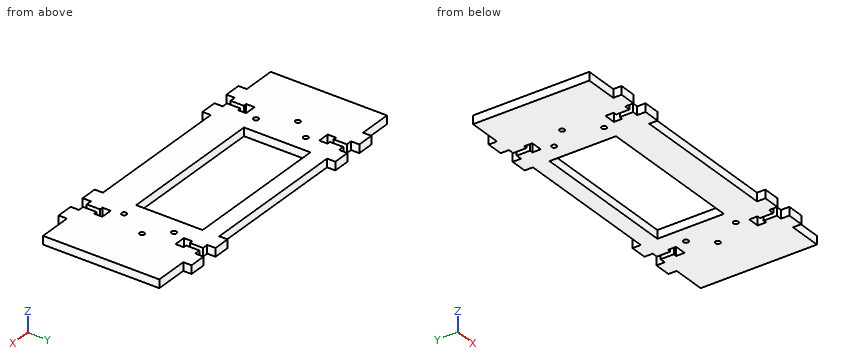
Autodesk Inventor part; units mm, degrees
ref_plane "YZ Plane" through (0, 0, 0) normal (1, 0, 0) x (0, 1, 0)
ref_plane "XZ Plane" through (0, 0, 0) normal (0, 1, 0) x (-1, 0, 0)
ref_plane "XY Plane" through (0, 0, 0) normal (0, 0, 1) x (1, 0, 0)
sketch "Sketch1" plane through (0, 0, 0) normal (0, 0, 1) x (1, 0, 0)
  line L0 (0, 0) -> (190, 0)
  line L1 (190, 0) -> (190, -70)
  line L2 (190, -70) -> (0, -70)
  line L3 (0, -70) -> (0, 0)
  line L4 (0, 0) -> (0, -40)
  line L5 (0, 0) -> (0, -10)
  line L6 (50, -10) -> (50, -50)
  line L7 (50, -50) -> (140, -50)
  line L8 (140, -50) -> (140, -10)
  line L9 (140, -10) -> (50, -10)
  circle A0 centre (40, -20) radius 1.5
  circle A1 centre (150, -20) radius 1.5
  circle A2 centre (150, -50) radius 1.5
  circle A3 centre (40, -50) radius 1.5
  line L10 (50, -10) -> (50, -12)
  line L11 (50, -12) -> (50, -32)
  line L12 (50, -32) -> (30, -32)
  line L13 (140, -32) -> (160, -32)
  circle A4 centre (30, -32) radius 1.5
  circle A5 centre (160, -32) radius 1.5
  dimension "d0" = 190
  dimension "d1" = 70
  dimension "d116" = 40
  dimension "d118" = 50
  dimension "d119" = 40
  dimension "d120" = 90
  dimension "d125" = 3
  dimension "d126" = 3
  dimension "d127" = 3
  dimension "d128" = 3
  dimension "d130" = 20
  dimension "d131" = 20
  dimension "d132" = 20
  dimension "d133" = 3
  dimension "d134" = 3
  dimension "d140" = 20
  dimension "d141" = 20
  dimension "d145" = 18
  dimension "d146" = 18
extrude "Extrusion3" add sketch "Sketch1" along normal blind 5 contours L0 L1 L2 L3 | L9 L8 L7 L6 | A5 | A4 | A0 | A1 | A2 | A3
sketch "Sketch3" plane through (0, 0, 0) normal (0, 0, -1) x (-1, 0, 0)
  line L0 (0, 0) -> (-35, 0)
  line L1 (-35, 0) -> (-35, -13)
  line L2 (-35, -13) -> (-31.5, -13)
  line L3 (-35, -13) -> (-38.5, -13)
  line L4 (-38.5, -13) -> (-38.5, -8)
  line L5 (-38.5, -8) -> (-36.5, -8)
  line L6 (-36.5, -8) -> (-36.5, 0)
  line L7 (-31.5, -13) -> (-31.5, -8)
  line L8 (-31.5, -8) -> (-33.5, -8)
  line L9 (-33.5, -8) -> (-33.5, 0)
  line L10 (-35, 0) -> (-75, 0) construction
  line L11 (-75, 0) -> (-75, -13)
  line L12 (-75, -13) -> (-71.5, -13)
  line L13 (-75, -13) -> (-78.5, -13)
  line L14 (-78.5, -13) -> (-78.5, -8)
  line L15 (-78.5, -8) -> (-76.5, -8)
  line L16 (-71.5, -13) -> (-71.5, -8)
  line L17 (-71.5, -8) -> (-73.5, -8)
  line L18 (-73.5, -8) -> (-73.5, 0)
  line L19 (-76.5, -8) -> (-76.5, 0)
  line L20 (0, 0) -> (-190, 0)
  line L21 (-75, 0) -> (-115, 0)
  line L22 (-115, 0) -> (-115, -13)
  line L23 (-115, -13) -> (-111.5, -13)
  line L24 (-111.5, -13) -> (-111.5, -8)
  line L25 (-111.5, -8) -> (-113.5, -8)
  line L26 (-113.5, -8) -> (-113.5, 0)
  line L27 (-115, -13) -> (-118.5, -13)
  line L28 (-118.5, -13) -> (-118.5, -8)
  line L29 (-118.5, -8) -> (-116.5, -8)
  line L30 (-116.5, -8) -> (-116.5, 0)
  line L31 (-115, 0) -> (-155, 0)
  line L32 (-155, 0) -> (-155, -13)
  line L33 (-155, -13) -> (-151.5, -13)
  line L34 (-151.5, -13) -> (-151.5, -8)
  line L35 (-151.5, -8) -> (-153.5, -8)
  line L36 (-153.5, -8) -> (-153.5, 0)
  line L37 (-155, -13) -> (-158.5, -13)
  line L38 (-158.5, -13) -> (-158.5, -8)
  line L39 (-158.5, -8) -> (-156.5, -8)
  line L40 (-156.5, -8) -> (-156.5, 0)
  line L41 (-76.5, 0) -> (-73.5, 0)
  line L42 (-33.5, -8) -> (-31.5, -8)
  line L43 (-36.5, 0) -> (-33.5, 0)
  line L44 (-155, 0) -> (-155, -70)
  line L45 (-115, 0) -> (-115, -70)
  line L46 (-75, 0) -> (-75, -70)
  line L47 (-35, 0) -> (-35, -70)
  line L48 (-155, -70) -> (-153.5, -70)
  line L49 (-153.5, -70) -> (-153.5, -62)
  line L50 (-153.5, -62) -> (-151.5, -62)
  line L51 (-151.5, -62) -> (-151.5, -57)
  line L52 (-151.5, -57) -> (-155, -57)
  line L53 (-155, -70) -> (-156.5, -70)
  line L54 (-156.5, -70) -> (-156.5, -62)
  line L55 (-156.5, -62) -> (-158.5, -62)
  line L56 (-158.5, -62) -> (-158.5, -57)
  line L57 (-158.5, -57) -> (-155, -57)
  line L58 (-115, -70) -> (-113.5, -70)
  line L59 (-113.5, -70) -> (-113.5, -62)
  line L60 (-113.5, -62) -> (-111.5, -62)
  line L61 (-111.5, -62) -> (-111.5, -57)
  line L62 (-111.5, -57) -> (-115, -57)
  line L63 (-115, -70) -> (-116.5, -70)
  line L64 (-116.5, -70) -> (-116.5, -62)
  line L65 (-116.5, -62) -> (-118.5, -62)
  line L66 (-118.5, -62) -> (-118.5, -57)
  line L67 (-118.5, -57) -> (-115, -57)
  line L68 (-75, -70) -> (-73.5, -70)
  line L69 (-73.5, -70) -> (-73.5, -62)
  line L70 (-73.5, -62) -> (-71.5, -62)
  line L71 (-71.5, -62) -> (-71.5, -57)
  line L72 (-71.5, -57) -> (-75, -57)
  line L73 (-75, -70) -> (-76.5, -70)
  line L74 (-76.5, -70) -> (-76.5, -62)
  line L75 (-76.5, -62) -> (-78.5, -62)
  line L76 (-78.5, -62) -> (-78.5, -57)
  line L77 (-78.5, -57) -> (-75, -57)
  line L78 (-35, -70) -> (-33.5, -70)
  line L79 (-33.5, -70) -> (-33.5, -62)
  line L80 (-33.5, -62) -> (-31.5, -62)
  line L81 (-31.5, -62) -> (-31.5, -57)
  line L82 (-31.5, -57) -> (-38.5, -57)
  line L83 (-38.5, -57) -> (-38.5, -62)
  line L84 (-38.5, -62) -> (-36.5, -62)
  line L85 (-36.5, -62) -> (-36.5, -70)
  line L86 (-36.5, -70) -> (-35, -70)
  dimension "d14" = 35
  dimension "d15" = 13
  dimension "d16" = 3.5
  dimension "d17" = 3.5
  dimension "d18" = 5
  dimension "d19" = 2
  dimension "d20" = 2
  dimension "d21" = 40
  dimension "d22" = 13
  dimension "d23" = 3.5
  dimension "d24" = 3.5
  dimension "d25" = 5
  dimension "d26" = 2
  dimension "d27" = 2
  dimension "d28" = 40
  dimension "d29" = 8
  dimension "d30" = 13
  dimension "d31" = 40
  dimension "d32" = 13
  dimension "d33" = 3.5
  dimension "d34" = 5
  dimension "d35" = 2
  dimension "d36" = 3.5
  dimension "d37" = 5
  dimension "d38" = 2
  dimension "d39" = 40
  dimension "d40" = 13
  dimension "d41" = 3.5
  dimension "d42" = 5
  dimension "d43" = 2
  dimension "d44" = 3.5
  dimension "d45" = 5
  dimension "d46" = 2
  dimension "d63" = 8
  dimension "d66" = 1.5
  dimension "d67" = 5
  dimension "d68" = 1.5
  dimension "d69" = 2
  dimension "d70" = 5
  dimension "d71" = 1.5
  dimension "d72" = 2
  dimension "d73" = 8
  dimension "d74" = 2
  dimension "d75" = 1.5
extrude "Extrusion4" cut sketch "Sketch3" against normal blind 5 contours L32 L37 L38 L39 L40 L20
extrude "Extrusion5" cut sketch "Sketch3" against normal blind 5 contours L36 L35 L34 L33 L32 L20
extrude "Extrusion9" cut sketch "Sketch3" against normal blind 5 contours L9 L8 L7 L2 L1 L0
extrude "Extrusion10" cut sketch "Sketch3" against normal blind 5 contours L1 L3 L4 L5 L6 L20
extrude "Extrusion11" cut sketch "Sketch3" against normal blind 5 contours L44 L53 L54 L55 L56 L57
extrude "Extrusion12" cut sketch "Sketch3" against normal blind 5 contours L52 L51 L50 L49 L48 L44
extrude "Extrusion17" cut sketch "Sketch3" against normal blind 5 contours L82 L81 L80 L79 L78 L47 | L47 L86 L85 L84 L83 L82
sketch "Sketch4" plane through (153.5, -70, 0) normal (0, -1, 0) x (1, 0, 0)
  line L0 (-153.5, 0) -> (-133.5, 0)
  line L1 (-133.5, 0) -> (-133.5, 5)
  line L2 (-133.5, 5) -> (-123.5, 5)
  line L3 (-123.5, 5) -> (-123.5, 0)
  line L4 (-123.5, 0) -> (-133.5, 0)
  line L5 (-123.5, 5) -> (-113.5, 5)
  line L6 (-113.5, 5) -> (-113.5, 0)
  line L7 (-113.5, 0) -> (-103.5, 0)
  line L8 (-103.5, 0) -> (-103.5, 5)
  line L9 (-103.5, 5) -> (-113.5, 5)
  line L10 (-153.5, 0) -> (36.5, 0)
  line L11 (36.5, 0) -> (16.5, 0)
  line L12 (16.5, 0) -> (16.5, 5)
  line L13 (16.5, 5) -> (6.5, 5)
  line L14 (6.5, 5) -> (6.5, 0)
  line L15 (6.5, 0) -> (-3.5, 0)
  line L16 (-3.5, 0) -> (-3.5, 5)
  line L17 (-3.5, 5) -> (-13.5, 5)
  line L18 (-13.5, 5) -> (-13.5, 0)
  dimension "d90" = 20
  dimension "d91" = 5
  dimension "d92" = 10
  dimension "d93" = 10
  dimension "d94" = 10
  dimension "d95" = 190
  dimension "d96" = 20
  dimension "d97" = 10
  dimension "d98" = 10
  dimension "d99" = 10
extrude "Extrusion18" add sketch "Sketch4" along normal blind 5 contours L14 L13 L12 L10 | L18 L17 L16 L10 | L1 L2 L3 L4 | L6 L9 L8 L7
sketch "Sketch5" plane through (190, 0, 5) normal (0, 1, 0) x (1, 0, 0)
  line L0 (-190, 5) -> (-170, 5)
  line L1 (-170, 5) -> (-170, 0)
  line L2 (-170, 0) -> (-160, 0)
  line L3 (-160, 0) -> (-160, 5)
  line L4 (-160, 5) -> (-170, 5)
  line L5 (-160, 5) -> (-150, 5)
  line L6 (-150, 5) -> (-150, 0)
  line L7 (-150, 0) -> (-140, 0)
  line L8 (-140, 0) -> (-140, 5)
  line L9 (-140, 5) -> (-150, 5)
  line L10 (-190, 5) -> (0, 5)
  line L11 (0, 5) -> (-20, 5)
  line L12 (-20, 5) -> (-20, 0)
  line L13 (-20, 0) -> (-30, 0)
  line L14 (-30, 0) -> (-30, 5)
  line L15 (-30, 5) -> (-40, 5)
  line L16 (-40, 5) -> (-40, 0)
  line L17 (-40, 0) -> (-50, 0)
  line L18 (-50, 0) -> (-50, 5)
  dimension "d102" = 20
  dimension "d103" = 5
  dimension "d104" = 10
  dimension "d105" = 10
  dimension "d106" = 10
  dimension "d107" = 190
  dimension "d108" = 20
  dimension "d109" = 5
  dimension "d110" = 10
  dimension "d111" = 10
  dimension "d112" = 5
  dimension "d113" = 10
extrude "Extrusion19" add sketch "Sketch5" along normal blind 5
extrude "Extrusion20" cut sketch "Sketch1" along normal blind 10 contours L9 L8 L7 L6
extrude "Extrusion22" cut sketch "Sketch1" along normal blind 10 contours A5 | A4 | A0 | A1 | A2 | A3
properties part number "lateral_mdf2"
Can you work these out from the model? Positions are in its coordinate system, mm. Round coordinates to 2 decimals unless told otherwise and drop trailing zeros. Order: outer loops, then holes, each group sorted by start corner. A loop starts at its lowest first (then second) coordinate and runs counter-clockwise, first axis right, second up. Notation, with made-up numbers: (-21, -26) - (18, -26) arc R18 cw to (18, -15) - close; hole circle Ø5 at (18.5, 67.5). An arc over 180 degrees is marked (long way). Answer in a Markdown table with one row per item.
(1) Please list where these lines run through material, in increasing order: L1, parallel to X at y = -32, z = 1.1; L2, parallel to X at y = -4, z = 2.5; L3, parallel to X at y = -60, z = 0.95. Write a range as from..to.
From the geometry:
| item | result |
|---|---|
| L1 | x = 0..28.5, 31.5..50, 140..158.5, 161.5..190 |
| L2 | x = 0..33.5, 36.5..153.5, 156.5..190 |
| L3 | x = 0..31.5, 38.5..151.5, 158.5..190 |
(2) Suppose I cut it at B-B, the plane x = 57. Please give me the cut outline in (y, z).
From the geometry:
| item | result |
|---|---|
| outline | (-70, 0) - (-50, 0) - (-50, 5) - (-70, 5) - close; (-10, 0) - (0, 0) - (0, 5) - (-10, 5) - close |
(3) Suppose I cut it at C-C, the plane y = -45. Please give me the cut outline in (x, z), plus the area to 3 significant figures.
From the geometry:
| item | result |
|---|---|
| outline | (0, 0) - (50, 0) - (50, 5) - (0, 5) - close; (140, 0) - (190, 0) - (190, 5) - (140, 5) - close |
| area | 500 mm2 |
(4) Suppose I cut it at A-A, the plane y = -3. Please give me the cut outline in (x, z), plus the area to 3 significant figures.
From the geometry:
| item | result |
|---|---|
| outline | (0, 0) - (33.5, 0) - (33.5, 5) - (0, 5) - close; (36.5, 0) - (153.5, 0) - (153.5, 5) - (36.5, 5) - close; (156.5, 0) - (190, 0) - (190, 5) - (156.5, 5) - close |
| area | 920 mm2 |
(5) For P1, Ø2.5, axis at y = 3.5, z = 3.5, coming from the +X side; P2, Ø2.5, axis at x = 35, z = 1.5, coming from the +Y side; P3, Ø1.5, axis at y = -71.5, z = 1.5, coming from the -X side, each with a flat end and sliding along its axis, tell me the tip position at first contact or that it passes through.
From the geometry:
| item | result |
|---|---|
| P1 | stops at x = 170 |
| P2 | stops at y = -13 |
| P3 | stops at x = 20 |
(6) Suppose I cut it at D-D, the plane z = 1.9. Count the separate pieces of the cut face and the enclosed holes in it, plus the area to 3 significant figures.
From the geometry:
| item | result |
|---|---|
| separate pieces | 1 |
| enclosed holes | 7 |
| area | 9,820 mm2 |
